Geometry check sheet. Reference: the model listing, model coordinates, mm. A direction names the side the tool comes from. Give positions to 0.01 mm unless a question says otherwise; leave off trailing zeros. Order: outer loops, then holes, each group sorted by start corner. A loop starts at its lowest first (then second) coordinate and runs counter-clockwise, first axis right, second up.
from build123d import *

# Parameters (mm, degrees)
BOSS_EXTRUDE1_DEPTH           = 1.6764
F_2_5MM_DOWEL_HOLE1_OUTLINE_R = 1.25
F_2_5MM_DOWEL_HOLE1_DEPTH     = 1.6764
SKETCH4_R                     = 3.175
BOSS_EXTRUDE2_DEPTH           = 5.08
SKETCH5_R                     = 2.1209
BOSS_EXTRUDE3_DEPTH           = 12.7


# Read off the part's stored shape, not the designer's step: Ø2.5mm Dowel Hole1
with BuildPart() as part:
    # Sketch1 → Boss-Extrude1 (new body)
    with BuildSketch(Plane(origin=(0, 0, 0), x_dir=(1, 0, 0), z_dir=(0, 1, 0))):
        with BuildLine():
            Line((-5.08, -6.35), (5.08, -6.35))
            ThreePointArc((5.08, -6.35), (5.978025612, -5.978025612), (6.35, -5.08))
            Line((6.35, -5.08), (6.35, 5.08))
            ThreePointArc((6.35, 5.08), (5.978025612, 5.978025612), (5.08, 6.35))
            Line((5.08, 6.35), (-5.08, 6.35))
            ThreePointArc((-5.08, 6.35), (-5.978025612, 5.978025612), (-6.35, 5.08))
            Line((-6.35, 5.08), (-6.35, -5.08))
            ThreePointArc((-6.35, -5.08), (-5.978025612, -5.978025612), (-5.08, -6.35))
        make_face()
    extrude(amount=BOSS_EXTRUDE1_DEPTH)

    # Ø2.5mm Dowel Hole1 outline → Ø2.5mm Dowel Hole1 (cut)
    with BuildSketch(Plane(origin=(0, 0, 0), x_dir=(1, 0, 0), z_dir=(0, 1, 0))):
        with Locations((4.318, -4.318)):
            Circle(F_2_5MM_DOWEL_HOLE1_OUTLINE_R)
        with Locations((-4.318, 4.318)):
            Circle(F_2_5MM_DOWEL_HOLE1_OUTLINE_R)
        with Locations((-4.318, -4.318)):
            Circle(F_2_5MM_DOWEL_HOLE1_OUTLINE_R)
        with Locations((4.318, 4.318)):
            Circle(F_2_5MM_DOWEL_HOLE1_OUTLINE_R)
    extrude(amount=F_2_5MM_DOWEL_HOLE1_DEPTH, mode=Mode.SUBTRACT)

    # Sketch4 → Boss-Extrude2 (add)
    with BuildSketch(Plane(origin=(0, 1.6764, 0), x_dir=(1, 0, 0), z_dir=(0, 1, 0))):
        with Locations(Location((0, 0, 0), (0, 0, 270))):
            Circle(SKETCH4_R)
    extrude(amount=BOSS_EXTRUDE2_DEPTH)

    # Sketch5 → Boss-Extrude3 (add)
    with BuildSketch(Plane.XZ):
        with Locations(Location((0, 0, 0), (0, 0, 90))):
            Circle(SKETCH5_R)
    extrude(amount=BOSS_EXTRUDE3_DEPTH)


solid = part.part
Item 1: Draft check along X on faces 1 (the flat face through (0, 1, -6.35)), 2 (the flat face through (6.35, 1, 0)), 3 (the cylindrical face through (3.326, 0.826, 5.079)). Enter one of: released by +X, released by -X, zero draft, split by the parting line, or undercut.
Reported:
face 1: zero draft
face 2: released by +X
face 3: undercut
Item 2: Sectioned sample at B-B (x = 0). Enter the section's corners in (y, z) (3 decimals), and give its area (3 significant figures).
Reported:
outline: (-12.7, -2.121) - (0, -2.121) - (0, -6.35) - (1.676, -6.35) - (1.676, -3.175) - (6.756, -3.175) - (6.756, 3.175) - (1.676, 3.175) - (1.676, 6.35) - (0, 6.35) - (0, 2.121) - (-12.7, 2.121) - close
area: 107 mm2
Item 3: Sectioned sample at A-A (z = 0). Enter the section's corners in (x, y) (3 decimals), and give its area (3 significant figures).
Reported:
outline: (-6.35, 0) - (-2.121, 0) - (-2.121, -12.7) - (2.121, -12.7) - (2.121, 0) - (6.35, 0) - (6.35, 1.676) - (3.175, 1.676) - (3.175, 6.756) - (-3.175, 6.756) - (-3.175, 1.676) - (-6.35, 1.676) - close
area: 107 mm2
Item 4: Scan lines: L1, parallel to Y at x = 2.5, z = 5.5; L2, parallel to Y at x = 1.5, z = 2.25; L3, parallel to Z at x = 3.75, y = 1. Record each from-to range of solid material in increasing order.
Reported:
L1: y = 0 to 1.68
L2: y = 0 to 6.76
L3: z = -6.35 to -5.43, -3.2 to 3.2, 5.43 to 6.35
Item 5: Sectioned sample at C-C (y = 5). Enter the section's corners in (x, z) (3 decimals).
Reported:
outline: circle Ø6.35 at (0, 0)
Item 6: Gauge pin test, flat ends, axial feed: pin 1 (2 mm diameter, centred on y = -5.5, z = 0.5, fed in from +X); pin 2 (3 mm diameter, centred on x = 4.318, z = 4.318, fed in from +Y); pin 3 (4 mm diameter, centred on x = -1.5, y = -3, fed in from -Z). Record the tip position at first contact, or that the pin passes through.
Reported:
pin 1: stops at x = 2.12
pin 2: stops at y = 1.68
pin 3: stops at z = -2.12
Item 7: Sectioned sample at D-D (y = -1.5). Enter the section's corners in (x, z).
Reported:
outline: circle Ø4.24 at (0, 0)
Item 8: Set-up check for faces 4 (the cylindrical face through (1.291, -6.261, -1.683)), 5 (the flat face through (-2, 1.676, -3)), 6 (the flat face through (0, -12.7, 0)): record each of +Z, -Z, +X, -X, +Y, -Y from which the full face is reachable in a straight line by a thin tool's end or side.
Reported:
face 4: -Y
face 5: +Y
face 6: +Z, -Z, +X, -X, -Y
